CAD build for the part. Positions are in the model's coordinates, mm. Give positions to 0.01 mm unless a question says otherwise; leave off trailing zeros. Write each loop counter-clockwise with the first axis right and the second up, starting at its lowest first coordinate (ties: lowest second). Pieces come first, ordered by that corner, then holes. Notation, with made-up numbers: (86.5, 45) - (126.5, 45) arc R28 ccw to (126.5, 78) - close; hole circle Ø5 at (23.25, 42). An arc over 180 degrees is marked (long way). Write item = value, one per line. Start each with the question number.
```python
from build123d import *

# Parameters (mm, degrees)
SKETCH1_R           = 34.925
BOSS_EXTRUDE1_DEPTH = 12.7
SKETCH2_R           = 3.175
BOSS_EXTRUDE2_DEPTH = 130.4
SKETCH3_R           = 3.175
BOSS_EXTRUDE3_DEPTH = 151.5
SKETCH4_R           = 1
BOSS_EXTRUDE4_DEPTH = 151.5
SKETCH5_R           = 15.941442814
BOSS_EXTRUDE5_DEPTH = 3
SKETCH6_R           = 15.941442814
BOSS_EXTRUDE6_DEPTH = 3


with BuildPart() as part:
    # Sketch1 → Boss-Extrude1 (new body)
    with BuildSketch(Plane(origin=(0, 0, 0), x_dir=(1, 0, 0), z_dir=(0, 1, 0))):
        with Locations(Location((0, 0, 0), (0, 0, 270))):
            Circle(SKETCH1_R)
    extrude(amount=BOSS_EXTRUDE1_DEPTH)

    # Sketch2 → Boss-Extrude2 (add)
    with BuildSketch(Plane(origin=(0, 12.7, 0), x_dir=(1, 0, 0), z_dir=(0, 1, 0))):
        with Locations(Location((-6.35, 6.35, 0), (0, 0, 270))):
            Circle(SKETCH2_R)
        with Locations(Location((6.35, 6.35, 0), (0, 0, 90))):
            Circle(SKETCH2_R)
        with Locations(Location((6.35, -6.35, 0), (0, 0, 270))):
            Circle(SKETCH2_R)
        with Locations(Location((-6.35, -6.35, 0), (0, 0, 90))):
            Circle(SKETCH2_R)
    extrude(amount=BOSS_EXTRUDE2_DEPTH)

    # Sketch3 → Boss-Extrude3 (add)
    with BuildSketch(Plane(origin=(0, 143.1, 0), x_dir=(1, 0, 0), z_dir=(0, 1, 0))):
        with Locations(Location((-6.35, -6.35, 0), (0, 0, 90))):
            Circle(SKETCH3_R)
    extrude(amount=BOSS_EXTRUDE3_DEPTH)

    # Sketch4 → Boss-Extrude4 (add)
    with BuildSketch(Plane(origin=(0, 143.1, 0), x_dir=(1, 0, 0), z_dir=(0, 1, 0))):
        with Locations(Location((-6.35, 6.35, 0), (0, 0, 270))):
            Circle(SKETCH4_R)
        with Locations(Location((6.35, 6.35, 0), (0, 0, 90))):
            Circle(SKETCH4_R)
        with Locations(Location((6.35, -6.35, 0), (0, 0, 270))):
            Circle(SKETCH4_R)
    extrude(amount=BOSS_EXTRUDE4_DEPTH)

    # Sketch5 → Boss-Extrude5 (add)
    with BuildSketch(Plane(origin=(0, 143.1, 0), x_dir=(1, 0, 0), z_dir=(0, 1, 0))):
        with Locations(Location((0, 0, 0), (0, 0, 270))):
            Circle(SKETCH5_R)
    extrude(amount=-BOSS_EXTRUDE5_DEPTH)

    # Sketch6 → Boss-Extrude6 (add)
    with BuildSketch(Plane(origin=(0, 294.6, 0), x_dir=(1, 0, 0), z_dir=(0, 1, 0))):
        with Locations(Location((0, 0, 0), (0, 0, 270))):
            Circle(SKETCH6_R)
    extrude(amount=-BOSS_EXTRUDE6_DEPTH)


solid = part.part
```
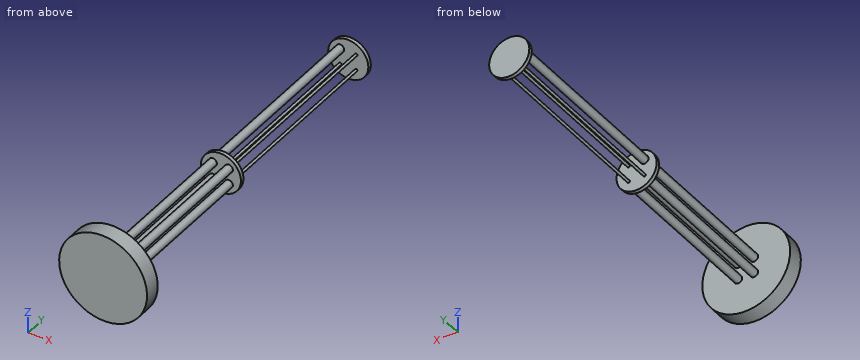
1. Cut at C-C (y = 67). Give the cut face in (x, z) (3 decimals).
2. Cut at D-D (y = 203). Give the cut face in (x, z) (3 decimals).
3. Cut at B-B (z = 0). Give the cut face in (x, y) (3 decimals), then the cut area to 3 significant figures.
4. Pin check, flat tips, straight feed: pin 1 Ø1 at (x, y) = (-4, 102) entering from -Z; pin 2 Ø6 at (x, y) = (3.5, 44.5) entering from -Z (3 decimals). Stop position of each tip, or through.
5. Cut at A-A (x = 0). Give the cut face in (y, z) (3 decimals).
6. Wall check: line 1 along Y through (x, z) = (1, 10.5); line 2 along X through (y, z) = (170.5, -6.5); line 3 along X through (y, z) = (117, 6). Give the ranges that are in metal, low to high.
Output:
q1.outline = circle Ø6.35 at (-6.35, -6.35); circle Ø6.35 at (-6.35, 6.35); circle Ø6.35 at (6.35, -6.35); circle Ø6.35 at (6.35, 6.35)
q2.outline = circle Ø6.35 at (-6.35, 6.35); circle Ø2 at (-6.35, -6.35); circle Ø2 at (6.35, -6.35); circle Ø2 at (6.35, 6.35)
q3.outline = (-34.925, 0) - (34.925, 0) - (34.925, 12.7) - (-34.925, 12.7) - close; (-15.941, 140.1) - (15.941, 140.1) - (15.941, 143.1) - (-15.941, 143.1) - close; (-15.941, 291.6) - (15.941, 291.6) - (15.941, 294.6) - (-15.941, 294.6) - close
q3.area = 1,080 mm2
q4.pin_1 = -8.93
q4.pin_2 = -9.525
q5.outline = (0, -34.925) - (12.7, -34.925) - (12.7, 34.925) - (0, 34.925) - close; (140.1, -15.941) - (143.1, -15.941) - (143.1, 15.941) - (140.1, 15.941) - close; (291.6, -15.941) - (294.6, -15.941) - (294.6, 15.941) - (291.6, 15.941) - close
q6.line_1 = 0 to 12.7, 140.1 to 143.1, 291.6 to 294.6
q6.line_2 = -7.34 to -5.36, 5.36 to 7.34
q6.line_3 = -9.51 to -3.19, 3.19 to 9.51
